The listing builds one solid part. Answer for the finished solid, in the listing's coordinates (mm). Give positions to 0.01 mm unless a question says otherwise; leave off trailing zeros. Write each loop counter-clockwise with the first axis right and the second up, starting at its lowest first coordinate (ties: lowest second). Pieces come first, ordered by that corner, then holes. Notation, with made-up numbers: (36.25, 74.5) - (52.25, 74.5) arc R29 cw to (52.25, 112.5) - close; hole circle Ø5 at (-3.5, 30.25). An arc over 180 degrees is marked (long way). Return JSON: item names as keys, results as strings.
from build123d import *

# Parameters (mm, degrees)
SKETCH2_R                  = 14.2875
SKETCH2_R_2                = 2.4892
BOSS_EXTRUDE1_DEPTH        = 3.175
F_9_0_196_DIAMETER_HOLE1_D = 4.9784


with BuildPart() as part:
    # Sketch2 → Boss-Extrude1 (new body)
    with BuildSketch(Plane.YZ):
        with BuildLine():
            Line((-29.326675554, -4.183509014), (35.011739717, -62.909380508))
            ThreePointArc((35.011739717, -62.909380508), (85.021103942, -53.236877748), (61.408883727, -8.104219103))
            Line((61.408883727, -8.104219103), (-24.617425063, 5.593731781))
            ThreePointArc((-24.617425063, 5.593731781), (-30.611222597, 2.457934521), (-29.326675554, -4.183509014))
        make_face()
        with Locations(Location((56.416233929, -39.459217876, 0), (0, 0, 270))):
            Circle(SKETCH2_R, mode=Mode.SUBTRACT)
        with Locations(Location((-25.508113787, 0, 0), (0, 0, 270))):
            Circle(SKETCH2_R_2, mode=Mode.SUBTRACT)
    extrude(amount=BOSS_EXTRUDE1_DEPTH)

    # #9 (0.196) Diameter Hole1 (through all)
    with Locations(Plane.YZ.offset(3.175)):
        with Locations((81.816233929, -39.459217876), (74.376746171, -57.419730118), (31.016233929, -39.459217876), (38.455721687, -21.498705633)):
            Hole(F_9_0_196_DIAMETER_HOLE1_D / 2)


solid = part.part
Item 1: A cutting plane is placed at C-C on z = 0. Determine the outline of the cut face in (x, y) (1 decimal), then the cut area to 3 significant figures.
Answer below:
{"outline": "(0, -31.2) - (3.2, -31.2) - (3.2, -28) - (0, -28) - close; (0, -23) - (3.2, -23) - (3.2, 10.5) - (0, 10.5) - close", "area": "117 mm²"}
Item 2: A cutting plane is placed at A-A on z = -50.5. Determine the outline of the cut face in (x, y) (3 decimals).
Answer below:
{"outline": "(0, 21.416) - (3.175, 21.416) - (3.175, 47.348) - (0, 47.348) - close; (0, 65.485) - (3.175, 65.485) - (3.175, 86.185) - (0, 86.185) - close"}
Item 3: A cutting plane is placed at B-B on x = 1.25. Give the number of separate pieces and of enclosed holes in the cut face, then the cut area to 3 significant figures.
Answer below:
{"separate pieces": "1", "enclosed holes": "6", "area": "4,440 mm²"}
Item 4: The mould has two halves that part along Y. Classify faces 1 (the face through (1.57, 19, -1.35)), 2 (the face through (1.6, 84.3, -39.3)), 3 (the face through (0, 41, -32)): +Y half, -Y half, draft (parallel to the pull), parting line (faces both ways), or undercut.
Answer below:
{"face 1": "+Y half", "face 2": "undercut", "face 3": "draft"}
Item 5: A flat-ended cylindrical pin translates along its axis: P1, Ø3, axis at y = 38.46, z = -21.5, coming from the -X side. Find the tip coordinate at first contact, or state that the pin passes through.
Answer below:
{"P1": "passes through"}
Item 6: Consider L1, parallel to Y at x = 2.95, z = -21.5; L2, parallel to Z at x = 0.2, y = 62; L3, parallel to Z at x = 2.9, y = 65. Determine where each line is inside the solid, lowest interval first.
Answer below:
{"L1": "y = -10.36 to 35.97, 40.94 to 82.6", "L2": "z = -70.71 to -52.61, -26.31 to -8.2", "L3": "z = -70.03 to -50.88, -28.04 to -8.89"}
Item 7: A cutting plane is placed at D-D on y = -10. Determine the outline of the cut face in (x, z) (3 decimals), then the cut area to 3 significant figures.
Answer below:
{"outline": "(0, -21.824) - (3.175, -21.824) - (3.175, 3.266) - (0, 3.266) - close", "area": "79.7 mm²"}
